from build123d import *

# Parameters (mm, degrees)
F0_R     = 2.5
F1_DEPTH = 10


with BuildPart() as f1:
    # F0 (on Top) → F1 (new body)
    with BuildSketch(Plane.XY):
        with BuildLine():
            Line((0, 20), (0, 35))
            ThreePointArc((0, 35), (-5.139641441, 34.620573159), (-10.1678475726, 33.4905191919))
            ThreePointArc((-10.1678475726, 33.4905191919), (-17.4537155293, 32.7918602935), (-24.5030527862, 34.7613374775))
            ThreePointArc((-24.5030527862, 34.7613374775), (-33.9418390183, 33.2078803829), (-34.1772546288, 23.6450097903))
            ThreePointArc((-34.1772546288, 23.6450097903), (-32.6723351007, 17.5032995342), (-33.160041137, 11.1987352765))
            ThreePointArc((-33.160041137, 11.1987352765), (-33.458628369, 10.0963588308), (-33.819654198, 9.012823638))
            ThreePointArc((-33.819654198, 9.012823638), (-34.994848156, -0.6005019029), (-33.4905191919, -10.1678475726))
            ThreePointArc((-33.4905191919, -10.1678475726), (-32.7918602935, -17.4537155293), (-34.7613374775, -24.5030527862))
            ThreePointArc((-34.7613374775, -24.5030527862), (-33.2078803829, -33.9418390183), (-23.6450097903, -34.1772546288))
            Line((-23.6450097903, -34.1772546288), (-17.5740434932, -25.4020854569))
            ThreePointArc((-17.5740434932, -25.4020854569), (-23.2594177785, -20.2640007089), (-27.9671079942, -14.2174274252))
            ThreePointArc((-27.9671079942, -14.2174274252), (-28.3098834226, -13.75089028), (-28.5817235471, -13.2397593292))
            ThreePointArc((-28.5817235471, -13.2397593292), (-26.2736614667, -7.8567708386), (-21.0708003204, -10.5463714686))
            ThreePointArc((-21.0708003204, -10.5463714686), (-17.4350672969, -15.0731601026), (-13.1010093591, -18.936618624))
            Line((-13.1010093591, -18.936618624), (-11.3789397329, -16.447484019))
            ThreePointArc((-11.3789397329, -16.447484019), (-19.0912241669, 5.9602986343), (0, 20))
        make_face()
        with Locations((-28.2842712475, -28.2842712475)):
            Circle(F0_R, mode=Mode.SUBTRACT)
        with BuildLine():
            ThreePointArc((-13.2397593292, 28.5817235471), (-7.8567708386, 26.2736614667), (-10.5463714686, 21.0708003204))
            ThreePointArc((-10.5463714686, 21.0708003204), (-17.096723239, 15.3462606412), (-22.0329337989, 8.1830708377))
            ThreePointArc((-22.0329337989, 8.1830708377), (-22.2601624756, 7.6240701847), (-22.5688933039, 7.1056110472))
            ThreePointArc((-22.5688933039, 7.1056110472), (-27.9497329821, 6.0062080975), (-29.3563625566, 11.3150230056))
            ThreePointArc((-29.3563625566, 11.3150230056), (-22.869546271, 20.6253378904), (-14.2174274252, 27.9671079942))
            ThreePointArc((-14.2174274252, 27.9671079942), (-13.75089028, 28.3098834226), (-13.2397593292, 28.5817235471))
        make_face(mode=Mode.SUBTRACT)
        with Locations((-28.2842712475, 28.2842712475)):
            Circle(F0_R, mode=Mode.SUBTRACT)
        with BuildLine():
            ThreePointArc((9.012823638, 33.819654198), (4.5448929069, 34.7036590069), (0, 35))
            Line((0, 35), (0, 20))
            ThreePointArc((0, 20), (7.6536686473, 18.4775906502), (14.1421356237, 14.1421356237))
            ThreePointArc((14.1421356237, 14.1421356237), (18.4775906502, 7.6536686473), (20, 0))
            ThreePointArc((20, 0), (14.1421356237, -14.1421356237), (0, -20))
            Line((0, -20), (0, -35))
            ThreePointArc((0, -35), (5.139641441, -34.620573159), (10.1678475726, -33.4905191919))
            ThreePointArc((10.1678475726, -33.4905191919), (17.4537155293, -32.7918602935), (24.5030527862, -34.7613374775))
            ThreePointArc((24.5030527862, -34.7613374775), (33.9418390183, -33.2078803829), (34.1772546288, -23.6450097903))
            ThreePointArc((34.1772546288, -23.6450097903), (32.6723351007, -17.5032995342), (33.160041137, -11.1987352765))
            ThreePointArc((33.160041137, -11.1987352765), (33.458628369, -10.0963588308), (33.819654198, -9.012823638))
            ThreePointArc((33.819654198, -9.012823638), (34.994848156, 0.6005019029), (33.4905191919, 10.1678475726))
            ThreePointArc((33.4905191919, 10.1678475726), (32.7918602935, 17.4537155293), (34.7613374775, 24.5030527862))
            ThreePointArc((34.7613374775, 24.5030527862), (33.2078803829, 33.9418390183), (23.6450097903, 34.1772546288))
            ThreePointArc((23.6450097903, 34.1772546288), (17.5032995342, 32.6723351007), (11.1987352765, 33.160041137))
            ThreePointArc((11.1987352765, 33.160041137), (10.0963588308, 33.458628369), (9.012823638, 33.819654198))
        make_face()
        with Locations((28.2842712475, -28.2842712475)):
            Circle(F0_R, mode=Mode.SUBTRACT)
        with BuildLine():
            ThreePointArc((13.2397593292, -28.5817235471), (7.8567708386, -26.2736614667), (10.5463714686, -21.0708003204))
            ThreePointArc((10.5463714686, -21.0708003204), (17.096723239, -15.3462606412), (22.0329337989, -8.1830708377))
            ThreePointArc((22.0329337989, -8.1830708377), (22.2601624756, -7.6240701847), (22.5688933039, -7.1056110472))
            ThreePointArc((22.5688933039, -7.1056110472), (27.9497329821, -6.0062080975), (29.3563625566, -11.3150230056))
            ThreePointArc((29.3563625566, -11.3150230056), (22.869546271, -20.6253378904), (14.2174274252, -27.9671079942))
            ThreePointArc((14.2174274252, -27.9671079942), (13.75089028, -28.3098834226), (13.2397593292, -28.5817235471))
        make_face(mode=Mode.SUBTRACT)
        with BuildLine():
            ThreePointArc((21.0708003204, 10.5463714686), (18.8162828052, 13.5301163041), (16.2562788277, 16.2562788277))
            ThreePointArc((16.2562788277, 16.2562788277), (12.4255192438, 19.432285732), (8.1830708377, 22.0329337989))
            ThreePointArc((8.1830708377, 22.0329337989), (7.6240701847, 22.2601624756), (7.1056110472, 22.5688933039))
            ThreePointArc((7.1056110472, 22.5688933039), (6.0062080975, 27.9497329821), (11.3150230056, 29.3563625566))
            ThreePointArc((11.3150230056, 29.3563625566), (16.8273746655, 25.9546878233), (21.7805752556, 21.7805752556))
            ThreePointArc((21.7805752556, 21.7805752556), (25.0844366917, 18.1712647028), (27.9671079942, 14.2174274252))
            ThreePointArc((27.9671079942, 14.2174274252), (28.3098834226, 13.75089028), (28.5817235471, 13.2397593292))
            ThreePointArc((28.5817235471, 13.2397593292), (26.2736614667, 7.8567708386), (21.0708003204, 10.5463714686))
        make_face(mode=Mode.SUBTRACT)
        with BuildLine():
            ThreePointArc((30.7842712475, 28.2842712475), (29.2409798284, 25.9745724162), (26.5165042945, 26.5165042945))
            ThreePointArc((26.5165042945, 26.5165042945), (27.3275626665, 30.5939700787), (30.7842712475, 28.2842712475))
        make_face(mode=Mode.SUBTRACT)
        with BuildLine():
            ThreePointArc((-6.8404028665, -18.7938524157), (-9.1849045913, -17.7661905778), (-11.3789397329, -16.447484019))
            Line((-11.3789397329, -16.447484019), (-13.1010093591, -18.936618624))
            ThreePointArc((-13.1010093591, -18.936618624), (-10.7064161122, -20.587025905), (-8.1830708377, -22.0329337989))
            ThreePointArc((-8.1830708377, -22.0329337989), (-8.1100323796, -22.0571549298), (-8.0374733682, -22.0827765885))
            Line((-8.0374733682, -22.0827765885), (-6.8404028665, -18.7938524157))
        make_face()
        with BuildLine():
            ThreePointArc((-9.012823638, -33.819654198), (-4.5448929069, -34.7036590069), (0, -35))
            Line((0, -35), (0, -20))
            ThreePointArc((0, -20), (-2.5970816611, -19.8306622896), (-5.150184936, -19.3255166846))
            Line((-5.150184936, -19.3255166846), (-6.2363085662, -23.4010791347))
            ThreePointArc((-6.2363085662, -23.4010791347), (-5.5404506045, -26.8715840588), (-7.8711189882, -29.5355299322))
            Line((-7.8711189882, -29.5355299322), (-9.012823638, -33.819654198))
        make_face()
        with BuildLine():
            ThreePointArc((-5.150184936, -19.3255166846), (-5.7778055515, -19.1472442667), (-6.3992773009, -18.9485949354))
            Line((-6.3992773009, -18.9485949354), (-7.5333779836, -22.3067263997))
            ThreePointArc((-7.5333779836, -22.3067263997), (-7.315380073, -22.4310964856), (-7.1056110472, -22.5688933039))
            ThreePointArc((-7.1056110472, -22.5688933039), (-6.6394848179, -22.9521074021), (-6.2363085662, -23.4010791347))
            Line((-6.2363085662, -23.4010791347), (-5.150184936, -19.3255166846))
        make_face()
        with BuildLine():
            ThreePointArc((-11.1987352765, -33.160041137), (-10.0963588308, -33.458628369), (-9.012823638, -33.819654198))
            Line((-9.012823638, -33.819654198), (-7.8711189882, -29.5355299322))
            ThreePointArc((-7.8711189882, -29.5355299322), (-8.9477708121, -29.8152650544), (-10.0598273225, -29.7876750907))
            Line((-10.0598273225, -29.7876750907), (-11.1987352765, -33.160041137))
        make_face()
        with BuildLine():
            ThreePointArc((-23.6450097903, -34.1772546288), (-17.5032995342, -32.6723351007), (-11.1987352765, -33.160041137))
            Line((-11.1987352765, -33.160041137), (-10.0598273225, -29.7876750907))
            ThreePointArc((-10.0598273225, -29.7876750907), (-10.7054391121, -29.6244425953), (-11.3150230056, -29.3563625566))
            ThreePointArc((-11.3150230056, -29.3563625566), (-14.5278498189, -27.5111014909), (-17.5740434932, -25.4020854569))
            Line((-17.5740434932, -25.4020854569), (-23.6450097903, -34.1772546288))
        make_face()
        with BuildLine():
            ThreePointArc((-6.3992773009, -18.9485949354), (-6.6202922175, -18.8725125766), (-6.8404028665, -18.7938524157))
            Line((-6.8404028665, -18.7938524157), (-8.0374733682, -22.0827765885))
            ThreePointArc((-8.0374733682, -22.0827765885), (-7.7815607221, -22.1860517531), (-7.5333779836, -22.3067263997))
            Line((-7.5333779836, -22.3067263997), (-6.3992773009, -18.9485949354))
        make_face()
    extrude(amount=F1_DEPTH)


solid = f1.part
The model under review builds one solid part; all positions refer to its coordinate system, in mm. A direction names the side the tool comes from. Round coordinates to 2 decimals unless told otherwise and drop trailing zeros. Write each loop counter-clockwise with the first axis right and the second up, starting at its lowest first coordinate (ties: lowest second). Pieces come first, ordered by that corner, then holes. Notation, with made-up numbers: M 89.5,10 L 125.5,10 A23 cw 125.5,27 Z; hole C 73,15 d11. An arc over 180 degrees is marked long. Answer as CSV lines item,"result". Start each with the question number.
Q1. Consider section C-C, the plane y = 19. Give the boundary of the cut face in (x, z) (1 decimal), then the cut area to 3 significant figures.
Q2. Consider section A-A, the plane y = -13. Give the boundary of the cut face in (x, z), then the cut area to 3 significant figures.
Q3. The part is to be moulded in two halves that separate along X. For faces 3 (the face through (15, -15, 0)), 4 (the face through (-22.976, 20.507, 4.93)), 5 (the face through (35, 0, 5)), say which applies: +X half, -X half, draft (parallel to the pull), parting line (faces both ways), or undercut.
Q4. Clearance check with flat-ended pins moving along their axes: P1, Ø3, axis at x = -28.28, y = -28.28, coming from the +Z side; P2, Ø3, axis at x = 23, z = 1.5, coming from the -Y side; P3, Ø6, axis at y = -24.5, z = 2.5, coming from the +X side; P4, Ø6, axis at x = 5.5, z = 7, coming from the +Y side. State where each tip first meets the part, or that it passes through.
Q5. Consider section D-D, the plane z = 4. State how many separate pieces and enclosed holes the cut face has, then the cut area to 3 significant figures.
Q6. Wall thickness on line 1 along X through (y, z) = (-20.5, 7.5); line 2 along X through (y, z) = (6, 5.25); line 3 along Y through (x, z) = (-18, 4.75): over which ranges is each line inside the solid? List them lowest first.
Q7. Consider section B-B, the plane y = 3. Give the boundary of the cut face in (x, z).
Q8. Tool access review of faces 1 (the face through (17.351, -32.783, 4.93)), 2 (the face through (17.015, -15.437, 4.93)): name each direction out of +Z, -Z, +X, -X, +Y, -Y from which nothing blocks a thin tool from reaching the whole face with its end or side.
Result set:
1,outline,"M -32.9,0 L -24.3,0 L -24.3,10 L -32.9,10 Z; M -13.3,0 L -6.2,0 L -6.2,10 L -13.3,10 Z; M 6.2,0 L 13,0 L 13,10 L 6.2,10 Z; M 24.4,0 L 33,0 L 33,10 L 24.4,10 Z"
1,area,"310 mm²"
2,outline,"M -32.9,0 L -28.68,0 L -28.68,10 L -32.9,10 Z; M -19.25,0 L -15.2,0 L -15.2,10 L -19.25,10 Z; M 15.2,0 L 19.01,0 L 19.01,10 L 15.2,10 Z; M 28.43,0 L 32.81,0 L 32.81,10 L 28.43,10 Z"
2,area,"165 mm²"
3,face 3,"draft"
3,face 4,"undercut"
3,face 5,"+X half"
4,P1,"passes through"
4,P2,"stops at y = -34.76"
4,P3,"stops at x = 35.74"
4,P4,"stops at y = 34.91"
5,separate pieces,"1"
5,enclosed holes,"9"
5,area,"2,450 mm²"
6,line 1,"x = -33.3 to -23.04, -10.84 to 11.37, 22.98 to 33.15"
6,line 2,"x = -34.48 to -27.94, -23.74 to -19.08, 19.08 to 34.48"
6,line 3,"y = -32.72 to -25.08, -14.46 to -8.72, 8.72 to 14.29, 25.22 to 32.85"
7,outline,"M -34.87,0 L -19.77,0 L -19.77,10 L -34.87,10 Z; M 19.77,0 L 34.87,0 L 34.87,10 L 19.77,10 Z"
8,face 1,"+Z, -Z, -Y"
8,face 2,"+Z, -Z"
